Build history of the part. All positions in model axes, mm. Face numbers are marked on the shaded views. A direction names the side the tool comes from. Round coordinates to 2 decimals unless told otherwise and drop trailing zeros. Write each loop counter-clockwise with the first axis right and the second up, starting at its lowest first coordinate (ties: lowest second). Pieces come first, ordered by that corner, then holes.
Autodesk Inventor part; units mm, degrees
ref_plane "YZ Plane" through (0, 0, 0) normal (1, 0, 0) x (0, 1, 0)
ref_plane "XZ Plane" through (0, 0, 0) normal (0, 1, 0) x (-1, 0, 0)
ref_plane "XY Plane" through (0, 0, 0) normal (0, 0, 1) x (1, 0, 0)
sketch "Эскиз1" plane through (0, 0, 0) normal (0, 0, 1) x (1, 0, 0)
  line L0 (0, 0) -> (0, 20)
  line L1 (0, 0) -> (0, 24)
  line L2 (0, 0) -> (0, 30)
  line L3 (0, 30) -> (-75, 30)
  line L4 (-75, 30) -> (-75, 0)
  line L5 (-75, 0) -> (-51, 0)
  line L6 (-51, 0) -> (-51, 15)
  line L7 (-51, 15) -> (-34, 15)
  line L8 (-34, 15) -> (-34, 30)
  line L9 (-54, 27) -> (-39, 27)
  line L10 (-39, 27) -> (-39, 18)
  line L11 (-39, 18) -> (-54, 18)
  line L12 (-54, 18) -> (-54, 27)
  dimension "d20" = 30
  dimension "d21" = 75
  dimension "d22" = 24
  dimension "d23" = 15
  dimension "d24" = 17
revolve "Вращение1" add sketch "Эскиз1" angle 360 about axis through (0, 0, 0) along (0, 1, 0)
sketch "Эскиз2" plane through (0, 30, 0) normal (0, 1, 0) x (1, 0, 0)
  circle A0 centre (0, 0) radius 32
  circle A1 centre (0, 0) radius 69
  line L0 (0, 0) -> (41.7812, 49.7929)
  line L1 (0, 0) -> (65, 0) construction
  circle A2 centre (41.7812, 49.7929) radius 1.5
  line L2 (0, 0) -> (-32.5, 56.2917)
  line L3 (0, 0) -> (65, 0) construction
  circle A3 centre (-32.5, 56.2917) radius 1.5
  line L4 (0, 0) -> (-11.2871, -64.0125)
  line L5 (0, 0) -> (65, 0) construction
  circle A4 centre (-11.2871, -64.0125) radius 1.5
  dimension "d8" = 65
  dimension "d9" = 50
  dimension "d10" = 3
  dimension "d11" = 65
  dimension "d12" = 120
  dimension "d13" = 3
  dimension "d14" = 65
  dimension "d15" = 100
  dimension "d16" = 3
extrude "Выдавливание1" cut sketch "Эскиз2" against normal through all contours A2 | A3 | A4
sketch "Эскиз5" plane through (0, 0, 0) normal (0, 1, 0) x (-1, 0, 0)
  line L0 (0, 0) -> (-64, 0)
sketch "Эскиз4" plane through (0, 0, 0) normal (0, 1, 0) x (-1, 0, 0)
  circle A0 centre (-64, 0) radius 5
  circle A1 centre (-64, 0) radius 6
  point P0 (0, 0)
  dimension "d27" = 12
extrude "Выдавливание3" cut sketch "Эскиз4" along normal blind 1
hole "Отверстие1" at (64, 0, 0) direction (0, 1, 0) diameter 9.9 depth 23 tip angle 118 counterbore diameter 10 counterbore depth 22
sketch "Эскиз6" plane through (0, 0, 0) normal (0, 0, 1) x (1, 0, 0)
  line L0 (54, 18) -> (54, 27)
  line L1 (54, 22.5) -> (59, 20)
  line L2 (68.95, 23) -> (59.05, 23)
  line L3 (59, 1) -> (59, 22)
  line L4 (59, 20) -> (59, 16.2)
  line L5 (59, 1) -> (59, 22)
  line L6 (51.0864, 23.9568) -> (54, 22.5)
  line L7 (59, 16.2) -> (49.5664, 20.9168)
  line L8 (49.5664, 20.9168) -> (51.0864, 23.9568)
  line L9 (59, 20) -> (60.52, 19.24)
  line L10 (60.52, 19.24) -> (59, 16.2)
  line L11 (-54, 18) -> (54, 18)
  point P0 (0, 0)
  point P1 (54, 18.7)
  dimension "d40" = 3.8
revolve "Вращение2" cut sketch "Эскиз6" angle 360 about axis through (54, 22.5, 0) along (0.8944272, -0.4472136, 0)
pattern_circular "Круговой массив1" count 2 over 360 about axis through (0, 22.5, 0) along (0, -1, 0) of "Вращение2", "Выдавливание3", "Отверстие1"
properties part number "Корпус сальника" material "Чугун, серый"
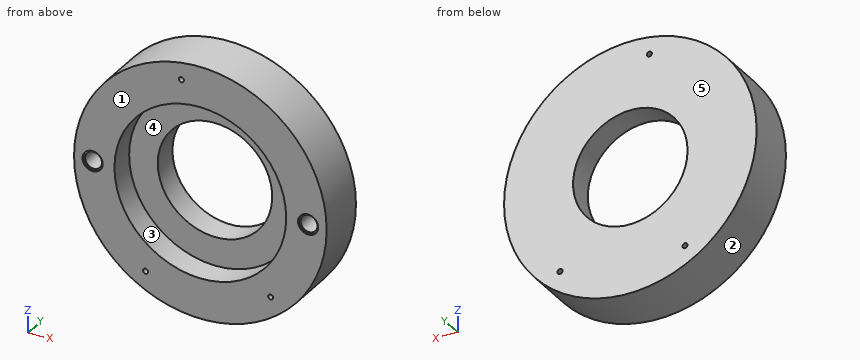
1) Slice it at A-A (x = 0). Write the cut outline in (y, z), plus the area to 3 significant figures.
Results:
outline: (0, -75) - (30, -75) - (30, -34) - (15, -34) - (15, -51) - (0, -51) - close; (0, 51) - (15, 51) - (15, 34) - (30, 34) - (30, 75) - (0, 75) - close; hole (18, -54) - (27, -54) - (27, -39) - (18, -39) - close; hole (18, 39) - (27, 39) - (27, 54) - (18, 54) - close
area: 1,680 mm2
2) Slice it at C-C (y = 10.25). Write the cut outline in (x, z).
Results:
outline: circle Ø150 at (0, 0); hole circle Ø10 at (-64, 0); hole circle Ø102 at (0, 0); hole circle Ø3 at (-32.5, -56.29); hole circle Ø3 at (-11.29, 64.01); hole circle Ø3 at (41.78, -49.79); hole circle Ø10 at (64, 0)
3) Mould opens along X. For the marked faces 1, 2 and 3 say: released by +X, released by -X, zero draft, split by the parting line, or undercut.
Results:
face 1: zero draft
face 2: split by the parting line
face 3: undercut
4) Slice it at B-B (z = -23). Write the cut outline in (x, y).
Results:
outline: (-71.39, 0) - (-45.52, 0) - (-45.52, 15) - (-25.04, 15) - (-25.04, 30) - (-71.39, 30) - close; (25.04, 15) - (45.52, 15) - (45.52, 0) - (71.39, 0) - (71.39, 30) - (25.04, 30) - close; hole (-48.86, 18) - (-31.5, 18) - (-31.5, 27) - (-48.86, 27) - close; hole (31.5, 18) - (48.86, 18) - (48.86, 27) - (31.5, 27) - close
5) Wall check: L1, parallel to X at y = 22.25, z = -22; L2, parallel to X at y = 21.25, z = 20; L3, parallel to Y at x = -23, z = -47. Give the ranges that are in metal, low to high.
Results:
L1: x = -71.7 to -49.32, -32.2 to -25.92, 25.92 to 32.2, 49.32 to 71.7
L2: x = -72.28 to -50.16, -33.48 to -27.5, 27.5 to 33.48, 50.16 to 72.28
L3: y = 0 to 18, 27 to 30
6) Pin check, flat tips, straight feed: pin 1 Ø19 at (x, z) = (-64, 0) entering from -Y; pin 2 Ø5 at (x, y) = (54.5, 23) entering from +Z; pin 3 Ø3 at (x, z) = (-63, 1) entering from -Y; pin 4 Ø1.5 at (x, y) = (16.5, 26.5) entering from +Z. Stop position of each tip, or through.
Results:
pin 1: stops at y = 0
pin 2: stops at z = 54.05
pin 3: stops at y = 24.22
pin 4: stops at z = 73.33
7) Which spindle directions (+Z, -Z, +X, -X, +Y, -Y) get a long thin tool onto all of the face, cutting with end or side? Do the marked faces 4 and 5. Say none if no direction does.
Results:
face 4: -Y
face 5: +Z, -Z, +X, -X, +Y
